Verification items for the finished model (mm, model axes). A direction names the side the tool comes from. Coordinates: 2 decimals unless noted, no trailing zeros. Loops run counter-clockwise (first coordinate to the right, second up) from the corner with the lowest first, then second, coordinate; pieces in that order, holes last.
Q1. Sectioned sample at D-D (y = 10.25). Count the separate pieces of the cut face and the enclosed holes in it, then the cut area to 3 significant figures.
Q2. Sectioned sample at C-C (x = -25.5). Enter the section's corners in (y, z).
Q3. Sectioned sample at A-A (y = 14.25). Enter the section's corners in (x, z), then the cut area to 3 significant figures.
Q4. Material ranges on probe 1 along X at (y, z) = (7.25, -11); probe 2 along Z at (x, y) = (27.5, 3.5); probe 3 along X at (y, z) = (10.5, 18.5), recorded low to high.
Q5. Mould release check, pull along X, two halves, no side actions. Record for faces 1 (the face through (-33.621, 10, -21)), 2 (the face through (-37, 17, 23)), 3 (the face through (-37.621, 2.7, 5.7)): +X half, -X half, draft (parallel to the pull), parting line (faces both ways), or undercut.
Q6. Sectioned sample at B-B (z = 18). Enter the section's corners in (x, y).
Q7. Access from +Z, -Z, +X, -X, +Y, -Y to the whole of each face (thin tool, end or side, straight path). Record for faces 4 (the face through (27.379, 10, -21)), 5 (the face through (-12.946, 1.521, 22.555)), 6 (the face through (-35, 10, -19.909)), 7 (the face through (34, 10, 20.091)).
Q8. Go/stop test with flat-tipped pins: P1, Ø4, axis at x = 19, z = -5, coming from the +Y side; P2, Ø10, axis at x = 6, y = 5, coming from the +Z side. Record where each tip stops, or that it passes through.
```python
from build123d import *

# Parameters (mm, degrees)
SKETCH1_W               = 73
SKETCH1_H               = 56
BOSS_EXTRUDE1_DEPTH     = 3
SKETCH2_R               = 1.5
CUT_EXTRUDE1_DEPTH      = 4
SKETCH4_W               = 2
SKETCH4_H               = 12
SKETCH4_H_2             = 19
SKETCH4_W_2             = 8
SKETCH4_H_3             = 2
BOSS_EXTRUDE2_DEPTH     = 14
SKETCH5_R               = 1.5
CUT_EXTRUDE2_DEPTH      = 4
SKETCH7_R               = 1.5
CUT_EXTRUDE4_DEPTH      = 1
CUT_EXTRUDE4_DEPTH_BACK = 74


with BuildPart() as part:
    # Sketch1 → Boss-Extrude1 (new body)
    with BuildSketch(Plane(origin=(0, 0, 0), x_dir=(1, 0, 0), z_dir=(0, 1, 0))):
        with Locations((-1.12052506, -6.090692124)):
            Rectangle(SKETCH1_W, SKETCH1_H)
    extrude(amount=BOSS_EXTRUDE1_DEPTH)

    # Sketch2 → Cut-Extrude1 (cut, through all)
    with BuildSketch(Plane(origin=(0, 3, 0), x_dir=(1, 0, 0), z_dir=(0, 1, 0))):
        with Locations((-12.62052506, 8.909307876)):
            Circle(SKETCH2_R)
        with Locations((-12.62052506, -21.090692124)):
            Circle(SKETCH2_R)
        with Locations((17.37947494, -21.090692124)):
            Circle(SKETCH2_R)
        with Locations((17.37947494, 8.909307876)):
            Circle(SKETCH2_R)
    extrude(amount=-CUT_EXTRUDE1_DEPTH, mode=Mode.SUBTRACT)

    # Sketch4 → Boss-Extrude2 (add)
    with BuildSketch(Plane(origin=(0, 3, 0), x_dir=(1, 0, 0), z_dir=(0, 1, 0))):
        Polygon((-33.62052506, 21.909307876), (-37.62052506, 21.909307876), (-37.62052506, 19.909307876), (-35.62052506, 19.909307876), (-33.62052506, 19.909307876), align=None)
        Polygon((35.37947494, 21.909307876), (27.37947494, 21.909307876), (27.37947494, 19.909307876), (33.37947494, 19.909307876), (35.37947494, 19.909307876), align=None)
        with Locations((34.37947494, 13.909307876)):
            Rectangle(SKETCH4_W, SKETCH4_H)
        with Locations((34.37947494, -26.090692124)):
            Rectangle(SKETCH4_W, SKETCH4_H)
        Polygon((-35.62052506, -32.090692124), (-37.62052506, -32.090692124), (-37.62052506, -34.090692124), (-33.62052506, -34.090692124), (-33.62052506, -32.090692124), align=None)
        with Locations((-36.62052506, -22.590692124)):
            Rectangle(SKETCH4_W, SKETCH4_H_2)
        with Locations((-36.62052506, 10.409307876)):
            Rectangle(SKETCH4_W, SKETCH4_H_2)
        with Locations((31.37947494, -33.090692124)):
            Rectangle(SKETCH4_W_2, SKETCH4_H_3)
    extrude(amount=BOSS_EXTRUDE2_DEPTH)

    # Sketch5 → Cut-Extrude2 (cut, through all)
    with BuildSketch(Plane(origin=(0, 3, 0), x_dir=(1, 0, 0), z_dir=(0, 1, 0))):
        with Locations((30.87947494, 16.409307876)):
            Circle(SKETCH5_R)
        with Locations((30.87947494, -28.590692124)):
            Circle(SKETCH5_R)
        with Locations((-14.12052506, 16.409307876)):
            Circle(SKETCH5_R)
        with Locations((-14.12052506, -28.590692124)):
            Circle(SKETCH5_R)
    extrude(amount=-CUT_EXTRUDE2_DEPTH, mode=Mode.SUBTRACT)

    # Sketch7 → Cut-Extrude4 (cut, two sides)
    with BuildSketch(Plane(origin=(35.37947494, 0, 0), x_dir=(0, 0, -1), z_dir=(1, 0, 0))) as cut_extrude4_sk:
        with Locations((-27.090692124, 11)):
            Circle(SKETCH7_R)
        with Locations((14.909307876, 11)):
            Circle(SKETCH7_R)
    extrude(amount=CUT_EXTRUDE4_DEPTH, mode=Mode.SUBTRACT)
    extrude(cut_extrude4_sk.sketch, amount=-CUT_EXTRUDE4_DEPTH_BACK, mode=Mode.SUBTRACT)


solid = part.part
```
Geometry check:
1. separate pieces: 8
1. enclosed holes: 0
1. area: 151 mm2
2. outline: (0, -21.91) - (3, -21.91) - (3, 34.09) - (0, 34.09) - close
3. outline: (-37.62, -21.91) - (-33.62, -21.91) - (-33.62, -19.91) - (-35.62, -19.91) - (-35.62, -0.91) - (-37.62, -0.91) - close; (-37.62, 13.09) - (-35.62, 13.09) - (-35.62, 32.09) - (-33.62, 32.09) - (-33.62, 34.09) - (-37.62, 34.09) - close; (27.38, -21.91) - (35.38, -21.91) - (35.38, -7.91) - (33.38, -7.91) - (33.38, -19.91) - (27.38, -19.91) - close; (27.38, 32.09) - (33.38, 32.09) - (33.38, 20.09) - (35.38, 20.09) - (35.38, 34.09) - (27.38, 34.09) - close
3. area: 172 mm2
4. probe 1: x = -37.62 to -35.62, 33.38 to 35.38
4. probe 2: z = -21.91 to -19.91, 32.09 to 34.09
4. probe 3: x = -37.62 to -35.62
5. face 1: undercut
5. face 2: draft
5. face 3: -X half
6. outline: (-37.62, 0) - (35.38, 0) - (35.38, 3) - (-35.62, 3) - (-35.62, 17) - (-37.62, 17) - close
7. face 4: +Z, -Z, +Y
7. face 5: +Y, -Y
7. face 6: +Y
7. face 7: +X, +Y
8. P1: stops at y = 3
8. P2: stops at z = 34.09
